```python
from build123d import *

# Parameters (mm, degrees)
BOSS_EXTRUDE2_DEPTH = 1.5
BOSS_EXTRUDE4_DEPTH = 1.5
FILLET2_START       = -1.5
FILLET2_DEPTH       = 3
SKETCH4_R           = 2.5
BOSS_EXTRUDE5_DEPTH = 2
SKETCH7_W           = 3
SKETCH7_H           = 8.6
BOSS_EXTRUDE6_DEPTH = 10
SKETCH9_W           = 6.5
SKETCH9_H           = 8.6
BOSS_EXTRUDE7_DEPTH = 2
BOSS_EXTRUDE8_DEPTH = 3


with BuildPart() as part:
    # Sketch1 → Boss-Extrude2 (new body)
    with BuildSketch(Plane.XY):
        with BuildLine():
            Line((-10, 4.3), (10, 4.3))
            Line((10, 4.3), (10, -4.3))
            Line((10, -4.3), (-10, -4.3))
            ThreePointArc((-10, -4.3), (-5.7, 0), (-10, 4.3))
        make_face()
    boss_extrude2 = extrude(amount=BOSS_EXTRUDE2_DEPTH)

    # Sketch3 → Boss-Extrude4 (add)
    with BuildSketch(Plane.XY.offset(1.5)):
        with BuildLine():
            Line((7, 6.319539578), (7, -6.319539578))
            ThreePointArc((7, -6.319539578), (6.646374896, -7.082559561), (5.835601013, -7.305933502))
            Line((5.835601013, -7.305933502), (-7.164398987, -5.139266835))
            ThreePointArc((-7.164398987, -5.139266835), (-7.763019982, -4.799247808), (-8, -4.152872912))
            Line((-8, -4.152872912), (-8, 4.152872912))
            ThreePointArc((-8, 4.152872912), (-7.763019982, 4.799247808), (-7.164398987, 5.139266835))
            Line((-7.164398987, 5.139266835), (5.835601013, 7.305933502))
            ThreePointArc((5.835601013, 7.305933502), (6.646374896, 7.082559561), (7, 6.319539578))
        make_face()
    boss_extrude4 = extrude(amount=BOSS_EXTRUDE4_DEPTH)

    # Mirror1: Boss-Extrude2, Boss-Extrude4 across plane
    add(boss_extrude2.mirror(Plane(origin=(-10, 0, 0), x_dir=(1, 0, 0), z_dir=(0, 0, -1))))
    add(boss_extrude4.mirror(Plane(origin=(-10, 0, 0), x_dir=(1, 0, 0), z_dir=(0, 0, -1))))

    # Fillet2: read off the stored shape, not the designer's step
    # Fillet2 outline → Fillet2 (cut)
    with BuildSketch(Plane.XY.offset(FILLET2_START)):
        with BuildLine():
            Line((-10, -4.3), (-5.852711729, -4.3))
            ThreePointArc((-5.852711729, -4.3), (-6.753445183, -3.734372243), (-6.63521895, -2.677358491))
            ThreePointArc((-6.63521895, -2.677358491), (-8.132199356, -3.873153851), (-10, -4.3))
        make_face()
        with BuildLine():
            ThreePointArc((-10, 4.3), (-8.132199356, 3.873153851), (-6.63521895, 2.677358491))
            ThreePointArc((-6.63521895, 2.677358491), (-6.753445183, 3.734372243), (-5.852711729, 4.3))
            Line((-5.852711729, 4.3), (-10, 4.3))
        make_face()
    extrude(amount=FILLET2_DEPTH, mode=Mode.SUBTRACT)

    # Sketch4 → Boss-Extrude5 (add)
    with BuildSketch(Plane.XY.offset(3)):
        with Locations((-3, 0)):
            Circle(SKETCH4_R)
    extrude(amount=BOSS_EXTRUDE5_DEPTH)

    # Sketch7 → Boss-Extrude6 (add)
    with BuildSketch(Plane(origin=(10, 0, 0), x_dir=(0, 0, -1), z_dir=(1, 0, 0))):
        Rectangle(SKETCH7_W, SKETCH7_H)
    extrude(amount=BOSS_EXTRUDE6_DEPTH)

    # Sketch9 → Boss-Extrude7 (add)
    with BuildSketch(Plane.XY.offset(1.5)):
        with Locations((16.75, 0)):
            Rectangle(SKETCH9_W, SKETCH9_H)
    boss_extrude7 = extrude(amount=BOSS_EXTRUDE7_DEPTH)

    # Sketch10 → Boss-Extrude8 (add)
    with BuildSketch(Plane.XY.offset(3.5)):
        with BuildLine():
            ThreePointArc((8.401790779, 35.991921381), (1.457653493, 37.233388065), (0.183185936, 30.295231636))
            ThreePointArc((0.183185936, 30.295231636), (9.577117756, 0), (0.183185936, -30.295231636))
            ThreePointArc((0.183185936, -30.295231636), (1.457653493, -37.233388065), (8.401790779, -35.991921381))
            ThreePointArc((8.401790779, -35.991921381), (19.75, 0), (8.401790779, 35.991921381))
        make_face()
    boss_extrude8 = extrude(amount=BOSS_EXTRUDE8_DEPTH)

    # Mirror2: Boss-Extrude7, Boss-Extrude8 across plane
    add(boss_extrude7.mirror(Plane.XY))
    add(boss_extrude8.mirror(Plane.XY))


solid = part.part
```
Geometry check sheet. Reference: the model listing, model coordinates, mm. A direction names the side the tool comes from. Coordinates: 2 decimals unless noted, no trailing zeros. Order: outer loops, then holes, each group sorted by start corner. A loop starts at its lowest first (then second) coordinate and runs counter-clockwise, first axis right, second up. Notation, with made-up numbers: (8.25, -19.5) - (24.25, -19.5) arc R18 ccw to (24.25, -5.5) - close; hole circle Ø4 at (59, 49). An arc over 180 degrees is marked (long way). Answer in a Markdown table with one row per item. Add a question column.
1. Draft check along Y on faces 1 (the face through (20, 0, 0)), 2 (the face through (-0.8, 6.2, -2.2)), 3 (the face through (1.548, 37.295, -4.979)). Enter one of: +Y half, -Y half, draft (parallel to the pull), parting line (faces both ways), or undercut.
2. Access from +Z, -Z, +X, -X, +Y, -Y to the whole of each face (thin tool, end or side, straight path). Record for faces 4 (the face through (7, 0, 2)), 5 (the face through (10, 0, 1.5)), 6 (the face through (-0.57, -6.24, 2.24)).
3. Section check B-B (x = 4). Enter the section's corners in (y, z).
4. Section check A-A (y = -25.5). Enter the section's corners in (x, z).
5. Section check D-D (y = 0). Enter the section's corners in (x, z), plus the area to 3 significant figures.
6. Material ranges on L1, parallel to Z at x = 11.75, y = -1; L2, parallel to Z at x = 12, y = 20; L3, parallel to Y at x = 18, z = -2.5, recorded low to high. Write a range as [from, to].
7. Section check C-C (x = -3.5). Enter the section's corners in (y, z).
8. Gauge pin test, flat ends, axial feed: pin 1 Ø1 at (y, z) = (15.5, -5) entering from -X; pin 2 Ø16 at (x, y) = (4.5, -4.5) entering from -Z; pin 3 Ø4 at (x, y) = (-3.5, 0) entering from +Z; pin 4 Ø7.5 at (x, y) = (2, -2) entering from -Z. Record the tip position at first contact, or that the pin passes through.
Data:
| question | item | result |
|---|---|---|
| 1 | face 1 | draft |
| 1 | face 2 | +Y half |
| 1 | face 3 | undercut |
| 2 | face 4 | +Z, +Y, -Y |
| 2 | face 5 | +Y, -Y |
| 2 | face 6 | +Z, -Z, -X, -Y |
| 3 | outline | (-38.11, -6.5) - (-23.79, -6.5) - (-23.79, -3.5) - (-38.11, -3.5) - close; (-38.11, 3.5) - (-23.79, 3.5) - (-23.79, 6.5) - (-38.11, 6.5) - close; (-7, -3) - (7, -3) - (7, -1.5) - (4.3, -1.5) - (4.3, 1.5) - (7, 1.5) - (7, 3) - (-7, 3) - (-7, 1.5) - (-4.3, 1.5) - (-4.3, -1.5) - (-7, -1.5) - close; (23.79, -6.5) - (38.11, -6.5) - (38.11, -3.5) - (23.79, -3.5) - close; (23.79, 3.5) - (38.11, 3.5) - (38.11, 6.5) - (23.79, 6.5) - close |
| 4 | outline | (3.12, -6.5) - (14.34, -6.5) - (14.34, -3.5) - (3.12, -3.5) - close; (3.12, 3.5) - (14.34, 3.5) - (14.34, 6.5) - (3.12, 6.5) - close |
| 5 | outline | (-8, -3) - (7, -3) - (7, -1.5) - (13.5, -1.5) - (13.5, -3.5) - (9.58, -3.5) - (9.58, -6.5) - (19.75, -6.5) - (19.75, -3.5) - (20, -3.5) - (20, 3.5) - (19.75, 3.5) - (19.75, 6.5) - (9.58, 6.5) - (9.58, 3.5) - (13.5, 3.5) - (13.5, 1.5) - (7, 1.5) - (7, 3) - (-0.5, 3) - (-0.5, 5) - (-5.5, 5) - (-5.5, 3) - (-8, 3) - (-8, 1.5) - (-5.7, 1.5) - (-5.7, -1.5) - (-8, -1.5) - close |
| 5 | area | 219 mm² |
| 6 | L1 | z = [-6.5, -3.5], [-1.5, 1.5], [3.5, 6.5] |
| 6 | L2 | z = [-6.5, -3.5], [3.5, 6.5] |
| 6 | L3 | y = [-4.3, 4.3] |
| 7 | outline | (-5.75, -3) - (5.75, -3) - (5.75, -1.5) - (4.3, -1.5) - (4.3, 1.5) - (5.75, 1.5) - (5.75, 3) - (2.45, 3) - (2.45, 5) - (-2.45, 5) - (-2.45, 3) - (-5.75, 3) - (-5.75, 1.5) - (-4.3, 1.5) - (-4.3, -1.5) - (-5.75, -1.5) - close |
| 8 | pin 1 | stops at x = 7.13 |
| 8 | pin 2 | stops at z = -6.5 |
| 8 | pin 3 | stops at z = 5 |
| 8 | pin 4 | stops at z = -3 |
